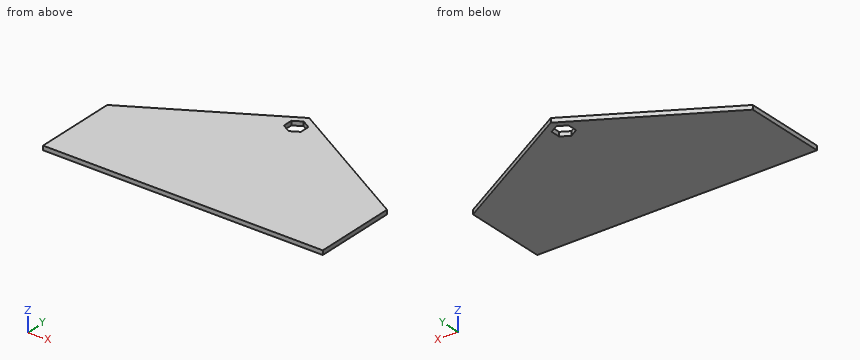
Autodesk Inventor part; units mm, degrees
ref_plane "YZ Plane" through (0, 0, 0) normal (1, 0, 0) x (0, 1, 0)
ref_plane "XZ Plane" through (0, 0, 0) normal (0, 1, 0) x (-1, 0, 0)
ref_plane "XY Plane" through (0, 0, 0) normal (0, 0, 1) x (1, 0, 0)
sketch "Sketch1" plane through (0, 0, 0) normal (0, 0, 1) x (1, 0, 0)
  line L0 (0, 0) -> (0, 201.9592)
  line L1 (0, 201.9592) -> (262.89, 353.7388)
  line L2 (262.89, 353.7388) -> (525.78, 201.9592)
  line L3 (525.78, 201.9592) -> (525.78, 0)
  line L4 (525.78, 0) -> (0, 0)
  point P0 (262.89, 0)
  dimension "d0" = 525.78
  dimension "d1" = 120
  dimension "d2" = 201.9592
extrude "Extrusion1" add sketch "Sketch1" along normal blind 6.35
sketch "Sketch3" plane through (0, 0, 6.35) normal (0, 0, 1) x (1, 0, 0)
  line L0 (50.8, 180.4886) -> (474.98, 180.4886)
  line L1 (474.98, 180.4886) -> (474.98, 50.8)
  line L2 (474.98, 50.8) -> (50.8, 50.8)
  line L3 (50.8, 50.8) -> (50.8, 180.4886)
  line L4 (0, 201.9592) -> (0, 0)
  line L5 (50.8, 180.4886) -> (262.89, 302.9388)
  line L6 (262.89, 302.9388) -> (474.98, 180.4886)
  line L7 (525.78, 0) -> (0, 0)
  line L8 (0, 201.9592) -> (0, 0)
  line L9 (0, 0) -> (525.78, 0)
  line L10 (525.78, 0) -> (525.78, 201.9592)
  line L11 (525.78, 201.9592) -> (262.89, 353.7388)
  line L12 (262.89, 353.7388) -> (0, 201.9592)
  point P0 (262.89, 180.4886)
  dimension "d15" = 120
  dimension "d16" = 50.8
  dimension "d17" = 50.8
  dimension "d18" = 50.8
extrude "Extrusion3" cut sketch "Sketch3" against normal through all
sketch "Sketch8" plane through (0, 0, 6.35) normal (0, 0, 1) x (1, 0, 0)
  line L0 (50.8, 50.8) -> (474.98, 50.8)
  line L1 (50.8, 180.4886) -> (50.8, 50.8)
  line L2 (50.8, 50.8) -> (474.98, 50.8)
  line L3 (474.98, 50.8) -> (474.98, 180.4886)
  line L4 (474.98, 180.4886) -> (262.89, 302.9388)
  line L5 (262.89, 302.9388) -> (50.8, 180.4886)
  line L6 (53.975, 178.6555) -> (53.975, 53.975)
  line L7 (53.975, 53.975) -> (471.805, 53.975)
  line L8 (471.805, 53.975) -> (471.805, 178.6555)
  line L9 (471.805, 178.6555) -> (262.89, 299.2727)
  line L10 (262.89, 299.2727) -> (53.975, 178.6555)
  point P0 (0, 0)
  dimension "d48" = 3.175
extrude "Extrusion8" cut sketch "Sketch8" against normal through all
sketch "Sketch9" plane through (0, 0, 6.35) normal (0, 0, 1) x (1, 0, 0)
  line L0 (262.89, 288.5374) -> (275.59, 281.205)
  line L1 (275.59, 281.205) -> (275.59, 266.5403)
  line L2 (275.59, 266.5403) -> (262.89, 259.208)
  line L3 (262.89, 259.208) -> (250.19, 266.5403)
  line L4 (250.19, 266.5403) -> (250.19, 281.205)
  line L5 (250.19, 281.205) -> (262.89, 288.5374)
  point P0 (0, 0)
  point P1 (262.89, 273.8727)
  point P2 (262.89, 299.2727)
  dimension "d51" = 25.4
  dimension "d52" = 25.4
extrude "Extrusion9" cut sketch "Sketch9" against normal through all
equation "\"d3\" = Panel_Thickness"
equation "\"Panel_Thickness\" = 6.35"
equation "\"Fit_Tolerance\" = 1.27"
equation "\"Tool_Dia\" = 6.35"
properties part number "BA15" material "Wood (Cherry)"
Build history of the part. All positions in model axes, mm. Coordinates: 2 decimals unless noted, no trailing zeros. Order: outer loops, then holes, each group sorted by start corner. A loop starts at its lowest first (then second) coordinate and runs counter-clockwise, first axis right, second up. Notation, with made-up numbers: M 84.5,-3.5 L 109.5,-3.5 A25 cw 109.5,26.5 Z; hole C 34.25,84 d10. An arc over 180 degrees is marked long. One line per question, with ' | ' between items. Start each with the question number.
Q1. Probe L1, parallel to Y at x = 250.5, z = 4.5 (3 decimals); L2, parallel to Y at x = 231.5, z = 5.5 (3 decimals); L3, parallel to Y at x = 253, z = 3.5 (3 decimals). List the from-to ranges inside material, lowest first. Write a range as from..to.
Q2. Saw through at A-A (z = 4.5). List the corners of the cut face in (x, y) (1 decimal), then the cut area to 3 significant figures.
Q3. Saw through at B-B (x = 123). List the corners of the cut face in (y, z) (3 decimals), then the cut area to 3 significant figures.
Q4. Flat gauge pins, fed straight in: pin 1 Ø3 at (y, z) = (275, 3.5) entering from +X; pin 2 Ø1.5 at (x, z) = (221, 2) entering from +Y; pin 3 Ø1.5 at (y, z) = (253, 2) entering from +X. Where does each tip first touch, or does it go through?
Q5. Saw through at C-C (y = 185). List the corners of the cut face in (x, z), then the cut area to 3 significant figures.
Check values:
1) L1: y = 53.975..266.361, 281.384..292.119 | L2: y = 53.975..281.15 | L3: y = 53.975..264.918, 282.827..293.563
2) outline: M 54,54 L 471.8,54 L 471.8,178.7 L 262.9,299.3 L 54,178.7 Z; hole M 250.2,266.5 L 262.9,259.2 L 275.6,266.5 L 275.6,281.2 L 262.9,288.5 L 250.2,281.2 Z | area: 76,700 mm2
3) outline: M 53.975,0 L 218.507,0 L 218.507,6.35 L 53.975,6.35 Z | area: 1,040 mm2
4) pin 1: stops at x = 307.53 | pin 2: stops at y = 275.52 | pin 3: stops at x = 344.34
5) outline: M 64.96,0 L 460.82,0 L 460.82,6.35 L 64.96,6.35 Z | area: 2,510 mm2
